Geometry: final body of the model. Coordinates: model frame, mm. Face numbers are marked on the shaded views. A direction names the side the tool comes from. Give positions to 0.01 mm unless a question says otherwise; leave off trailing zeros. Write each loop counter-clockwise with the first axis right and the second up, starting at its lowest first coordinate (ties: lowest second). Pieces come first, ordered by that corner, then holes.
Q1. Line query: L1, parallel to X at y = 3.75, z = 1; L2, parallel to Y at x = 20.6, z = -9; L3, parallel to Y at x = 20.3, z = 6.25. Output: solid intervals per line, ascending.
Q2. Draft query along Z for the marked faces 4, 5, 6 and 7. Return one class per face: pulls with the +Z half, pulls with the -Z half, needs draft (parallel to the pull), parting line crosses it, or undercut.
Q3. Cut plane D-D on z = -5.75. Return the cut outline in (x, y).
Q4. Pin query (flat end, axial travel): pin 1 (8.5 mm diameter, centred on x = 26.5, z = -0.5, fed in from +Y); pin 2 (0.8 mm diameter, centred on x = 20.5, z = 1.5, fed in from +Y). Return the tip coordinate at first contact, or that it passes through.
Q5. Reachability of the marked faces 1, 2 and 3 from +Z, -Z, +X, -X, +Y, -Y: full face, straight path, thin tool, end or side. Return the list, or none.
Q6. Cut plane A-A on y = 3.5. Return the cut outline in (x, z).
Q7. Cut plane C-C on x = 35.5. Return the cut outline in (y, z), plus the area to 3 significant figures.
Q8. Cut plane B-B on z = 7.5. Return the cut outline in (x, y).
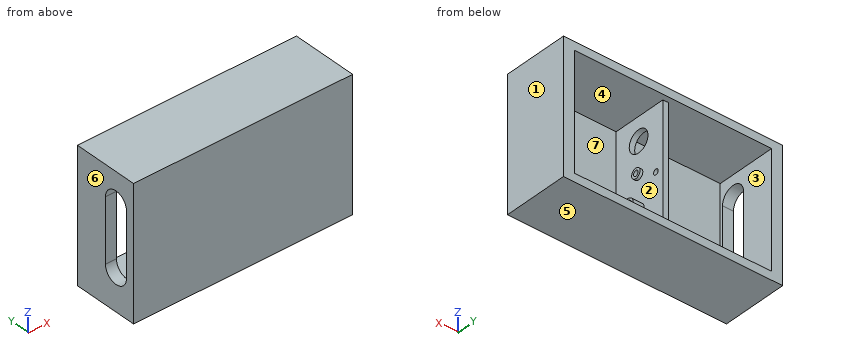
```python
from build123d import *

# Parameters (mm, degrees)
SKETCH_2_W               = 24
SKETCH_2_H               = 12
EXTRUDE_1_DEPTH          = 40
SKETCH_3_W               = 36
SKETCH_3_H               = 21
CUT_EXTRUDE_1_DEPTH      = 11
CUT_EXTRUDE_2_DEPTH      = 2
SKETCH_7_W               = 1
SKETCH_7_H               = 21
EXTRUDE_4_DEPTH          = 10
SKETCH_8_R               = 0.85
CUT_EXTRUDE_3_DEPTH      = 3
SKETCH_9_R               = 1.2
EXTRUDE_5_DEPTH          = 2
CUT_EXTRUDE_START        = -2
SKETCH_10_R              = 0.85
CUT_EXTRUDE_4_DEPTH      = 2
SKETCH_11_R              = 0.9
EXTRUDE_6_DEPTH          = 0.5
CUT_EXTRUDE_5_DEPTH      = 17
CUT_EXTRUDE_5_DEPTH_BACK = 2
SKETCH_12_R              = 0.5
SKETCH_13_R              = 2
CUT_EXTRUDE_6_DEPTH      = 2
SKETCH_14_R              = 0.5
CUT_EXTRUDE_7_DEPTH      = 2


with BuildPart() as part:
    # 草图2 → 凸台-拉伸1 (new body)
    with BuildSketch(Plane(origin=(0, 0, 0), x_dir=(0, 0, -1), z_dir=(1, 0, 0))):
        Rectangle(SKETCH_2_W, SKETCH_2_H)
    extrude(amount=EXTRUDE_1_DEPTH)

    # 草图3 → 切除-拉伸1 (cut)
    with BuildSketch(Plane(origin=(0, 6, 0), x_dir=(1, 0, 0), z_dir=(0, 1, 0))):
        with Locations((20, 0)):
            Rectangle(SKETCH_3_W, SKETCH_3_H)
    extrude(amount=-CUT_EXTRUDE_1_DEPTH, mode=Mode.SUBTRACT)

    # 草图4 → 切除-拉伸2 (cut)
    with BuildSketch(Plane.ZY):
        with BuildLine():
            Line((-5.05, 0), (6.45, 0))
            ThreePointArc((6.45, 0), (8.7, -2.25), (6.45, -4.5))
            Line((6.45, -4.5), (-5.05, -4.5))
            ThreePointArc((-5.05, -4.5), (-7.3, -2.25), (-5.05, 0))
        make_face()
    extrude(amount=-CUT_EXTRUDE_2_DEPTH, mode=Mode.SUBTRACT)

    # 草图7 → 凸台-拉伸4 (add)
    with BuildSketch(Plane(origin=(0, -5, 0), x_dir=(1, 0, 0), z_dir=(0, 1, 0))):
        with Locations((20.5, 0)):
            Rectangle(SKETCH_7_W, SKETCH_7_H)
    extrude(amount=EXTRUDE_4_DEPTH)

    # 草图8 → 切除-拉伸3 (cut)
    with BuildSketch(Plane.ZY.offset(-20)):
        with Locations((-5.7, -0.2)):
            Circle(SKETCH_8_R)
    extrude(amount=-CUT_EXTRUDE_3_DEPTH, mode=Mode.SUBTRACT)

    # 草图9 → 凸台-拉伸5 (add)
    with BuildSketch(Plane(origin=(21, 0, 0), x_dir=(0, 0, -1), z_dir=(1, 0, 0))):
        with Locations(Location((5.7, -0.2, 0), (0, 0, 180))):
            Circle(SKETCH_9_R)
    extrude(amount=EXTRUDE_5_DEPTH)

    # 草图10 → 切除-拉伸4 (cut)
    with BuildSketch(Plane(origin=(23, 0, 0), x_dir=(0, 0, -1), z_dir=(1, 0, 0)).offset(CUT_EXTRUDE_START)):
        with Locations(Location((5.7, -0.2, 0), (0, 0, 180))):
            Circle(SKETCH_10_R)
    extrude(amount=CUT_EXTRUDE_4_DEPTH, mode=Mode.SUBTRACT)

    # 草图11 → 凸台-拉伸6 (add)
    with BuildSketch(Plane(origin=(21, 0, 0), x_dir=(0, 0, -1), z_dir=(1, 0, 0))):
        with Locations(Location((-0.55, -0.2, 0), (0, 0, 180))):
            Circle(SKETCH_11_R)
    extrude(amount=EXTRUDE_6_DEPTH)

    # 草图12 → 切除-拉伸5 (cut, two sides: drawn at the far end of the back side and taken through both)
    with BuildSketch(Plane(origin=(21.5, 0, 0), x_dir=(0, 0, -1), z_dir=(1, 0, 0)).offset(-CUT_EXTRUDE_5_DEPTH_BACK)):
        with Locations((-0.55, -0.2)):
            Circle(SKETCH_12_R)
    extrude(amount=CUT_EXTRUDE_5_DEPTH + CUT_EXTRUDE_5_DEPTH_BACK, mode=Mode.SUBTRACT)

    # 草图13 → 切除-拉伸6 (cut)
    with BuildSketch(Plane(origin=(21, 0, 0), x_dir=(0, 0, -1), z_dir=(1, 0, 0))):
        with Locations((-6.25, -0.2)):
            Circle(SKETCH_13_R)
    extrude(amount=-CUT_EXTRUDE_6_DEPTH, mode=Mode.SUBTRACT)

    # 草图14 → 切除-拉伸7 (cut)
    with BuildSketch(Plane(origin=(21, 0, 0), x_dir=(0, 0, -1), z_dir=(1, 0, 0))):
        with Locations((9, -3.5)):
            Circle(SKETCH_14_R)
        with Locations((9, 3.5)):
            Circle(SKETCH_14_R)
        with Locations((1, 3.5)):
            Circle(SKETCH_14_R)
    extrude(amount=-CUT_EXTRUDE_7_DEPTH, mode=Mode.SUBTRACT)


solid = part.part
```
Data:
1. L1: x = 0 to 2, 20 to 21, 38 to 40
1. L2: y = -6 to -4, -3 to 3, 4 to 5
1. L3: y = -6 to -2.2, 1.8 to 5
2. face 4: undercut
2. face 5: pulls with the -Z half
2. face 6: needs draft
2. face 7: undercut
3. outline: (0, -6) - (40, -6) - (40, 6) - (38, 6) - (38, -5) - (21, -5) - (21, -1.4) - (23, -1.4) - (23, -1.05) - (20, -1.05) - (20, -5) - (2, -5) - (2, -4.39) - (0, -4.39) - close; (0, -0.11) - (2, -0.11) - (2, 6) - (0, 6) - close; (20, 0.65) - (23, 0.65) - (23, 1) - (21, 1) - (21, 5) - (20, 5) - close
4. pin 1: stops at y = -5
4. pin 2: stops at y = 5
5. face 1: +Z, -Z, +X, +Y, -Y
5. face 2: none
5. face 3: +Y
6. outline: (0, -12) - (40, -12) - (40, 12) - (0, 12) - close; (20, -8.5) - (21, -8.5) - (21, -1.5) - (20, -1.5) - close; hole (2, -10.5) - (20, -10.5) - (20, -9.5) - (21, -9.5) - (21, -10.5) - (38, -10.5) - (38, 10.5) - (21, 10.5) - (21, -0.5) - (20, -0.5) - (20, 10.5) - (2, 10.5) - close
7. outline: (-6, -12) - (6, -12) - (6, -10.5) - (-5, -10.5) - (-5, 10.5) - (6, 10.5) - (6, 12) - (-6, 12) - close
7. area: 57.0 mm2
8. outline: (0, -6) - (40, -6) - (40, 6) - (38, 6) - (38, -5) - (21, -5) - (21, -1.76) - (20, -1.76) - (20, -5) - (2, -5) - (2, -4.24) - (0, -4.24) - close; (0, -0.26) - (2, -0.26) - (2, 6) - (0, 6) - close; (20, 1.36) - (21, 1.36) - (21, 5) - (20, 5) - close
